```python
from build123d import *

# Parameters (mm, degrees)
SKETCH_1_W          = 470
SKETCH_1_H          = 510
SKETCH_1_H_2        = 20
SKETCH_1_W_2        = 20
EXTRUDE_1_DEPTH     = 12
SKETCH_2_W          = 185
SKETCH_2_H          = 153
SKETCH_2_W_2        = 20
SKETCH_2_H_2        = 20
CUT_EXTRUDE_1_DEPTH = 12


with BuildPart() as part:
    # ｽｹｯﾁ1 → ﾎﾞｽ - 押し出し1 (new body)
    with BuildSketch(Plane.XY):
        Rectangle(SKETCH_1_W, SKETCH_1_H)
        with Locations((0, 265)):
            Rectangle(SKETCH_1_W, SKETCH_1_H_2)
        with Locations((-245, 0)):
            Rectangle(SKETCH_1_W_2, SKETCH_1_H)
        with Locations((245, 0)):
            Rectangle(SKETCH_1_W_2, SKETCH_1_H)
        with Locations((0, -265)):
            Rectangle(SKETCH_1_W, SKETCH_1_H_2)
    extrude(amount=EXTRUDE_1_DEPTH)

    # ｽｹｯﾁ2 → ｶｯﾄ - 押し出し1 (cut)
    with BuildSketch(Plane(origin=(0, 0, 0), x_dir=(-1, 0, 0), z_dir=(0, 0, -1))):
        Polygon((-255, 255), (-235, 255), (-235, 275), (-50, 275), (-50, 308.587411224), (-364.697292758, 308.587411224), (-364.697292758, 102), (-255, 102), align=None)
        with Locations((-142.5, 178.5)):
            Rectangle(SKETCH_2_W, SKETCH_2_H)
        with Locations((-245, 178.5)):
            Rectangle(SKETCH_2_W_2, SKETCH_2_H)
        with Locations((-142.5, 265)):
            Rectangle(SKETCH_2_W, SKETCH_2_H_2)
    extrude(amount=-CUT_EXTRUDE_1_DEPTH, mode=Mode.SUBTRACT)


solid = part.part
```
Input: part model. Units: mm. Frame: model coordinates. A direction names the side the tool comes from. Coordinates: 2 decimals unless noted, no trailing zeros. Loops run counter-clockwise (first coordinate to the right, second up) from the corner with the lowest first, then second, coordinate; pieces in that order, holes last. Notation, with made-up numbers: (-20.75, -21.5) -> (7.25, -21.5) arc R21 ccw to (7.25, -11.5) -> close; hole circle Ø3 at (-10, 3.5). An arc over 180 degrees is marked (long way). Use a Markdown table: item, result.
1) Material intervals for line 1 along Y through (x, z) = (205, 9.5); line 2 along X through (y, z) = (163, 2), sorted ascending. Write a range as from..to.
Results found:
| item | result |
|---|---|
| line 1 | y = -275..102 |
| line 2 | x = -255..50 |
2) Cut plane C-C (x = 127). Return the cut outline in (y, z), then the cut area to 3 significant figures.
Results found:
| item | result |
|---|---|
| outline | (-275, 0) -> (102, 0) -> (102, 12) -> (-275, 12) -> close |
| area | 4,520 mm2 |
3) Contact query for flat-ended pins moving along their axis: pin 1 (12 mm diameter, centred on x = -146, y = 176.5, fed in from -Z); pin 2 (6 mm diameter, centred on x = 243, z = 8, fed in from -Y); pin 3 (6 mm diameter, centred on x = 144, z = 7.5, fed in from +Y); pin 4 (6 mm diameter, centred on y = -260, z = 9, fed in from -X). Output: stop coordinate, or through.
Results found:
| item | result |
|---|---|
| pin 1 | stops at z = 0 |
| pin 2 | stops at y = -255 |
| pin 3 | stops at y = 102 |
| pin 4 | stops at x = -235 |
4) Cut plane B-B (y = 167). Return the cut outline in (x, z), then the cut area to 3 significant figures.
Results found:
| item | result |
|---|---|
| outline | (-255, 0) -> (50, 0) -> (50, 12) -> (-255, 12) -> close |
| area | 3,660 mm2 |
5) Access query for faces 1 (the flat face through (-245, -255, 6)), 2 (the flat face through (-245, 255, 6)), 3 (the flat face through (50, 187, 6)), 4 (the flat face through (235, -265, 6)). Directions: +Z, -Z, +X, -X, +Y, -Y. A direction counts if a zero-diameter tool reaches every point of the face in a straight line with its end or side. Return the directions, or none.
Results found:
| item | result |
|---|---|
| face 1 | +Z, -Z, -X, -Y |
| face 2 | +Z, -Z, -X, +Y |
| face 3 | +Z, -Z, +X, +Y |
| face 4 | +Z, -Z, +X, -Y |
6) Cut plane A-A (z = 7.5). Return the cut outline in (x, y), then the cut area to 3 significant figures.
Results found:
| item | result |
|---|---|
| outline | (-255, -255) -> (-235, -255) -> (-235, -275) -> (235, -275) -> (235, -255) -> (255, -255) -> (255, 102) -> (50, 102) -> (50, 275) -> (-235, 275) -> (-235, 255) -> (-255, 255) -> close |
| area | 244,000 mm2 |
